The listing builds one solid part. Answer for the finished solid, in the listing's coordinates (mm). A direction names the side the tool comes from. Coordinates: 2 decimals unless noted, no trailing zeros. Order: outer loops, then holes, each group sorted by start corner. A loop starts at its lowest first (then second) coordinate and runs counter-clockwise, first axis right, second up. Notation, with made-up numbers: (43.25, 46.5) -> (90.25, 46.5) arc R19 cw to (90.25, 65.5) -> close; hole circle Ø2 at (20.5, 63.5). An arc over 180 degrees is marked (long way). Return JSON: item names as keys, results as strings.
Autodesk Inventor part; units mm, degrees
ref_plane "YZ Plane" through (0, 0, 0) normal (1, 0, 0) x (0, 1, 0)
ref_plane "XZ Plane" through (0, 0, 0) normal (0, 1, 0) x (-1, 0, 0)
ref_plane "XY Plane" through (0, 0, 0) normal (0, 0, 1) x (1, 0, 0)
sketch "Sketch1" plane through (0, 0, 0) normal (0, 1, 0) x (-1, 0, 0)
  line L0 (0, -14.7) -> (0, 14.7) construction
  line L1 (-13.4, 0) -> (33.15, 0) construction
  circle A0 centre (0, 0) radius 4.25
  circle A1 centre (16, 0) radius 7.975
  arc A2 (13.5391, -10.2075) -> (13.5391, 10.2075) centre (16, 0) ccw
  arc A3 (-1.582, 6.562) -> (-1.582, -6.562) centre (0, 0) ccw
  line L2 (13.5391, 10.2075) -> (-1.582, 6.562)
  line L3 (13.5391, -10.2075) -> (-1.582, -6.562)
  circle A4 centre (21, 0) radius 0.75
  circle A5 centre (11, 0) radius 0.75
  line L4 (16, 7.975) -> (16, -7.975) construction
  dimension "d0" = 8.5
  dimension "d1" = 15.95
  dimension "d2" = 16
  dimension "d3" = 21
  dimension "d4" = 13.5
  dimension "d5" = 1.5
  dimension "d6" = 1.5
  dimension "d7" = 10
extrude "Base" add sketch "Sketch1" along normal blind 3 contours A1 | L3 A3 L2 A2
extrude "Walls" add sketch "Sketch1" along normal blind 15 contours L3 A3 L2 A2
equation "\"d6\" = d5"
properties part number "transducer_holder" material "PC/ABS Plastic"
1. The part is cut by section B-B on x = -11. Give the vertices of the cut face in (y, z), and give its area (3 significant figures).
Answer block:
{"outline": "(0, -9.6) -> (15, -9.6) -> (15, -6.21) -> (3, -6.21) -> (3, -0.75) -> (0, -0.75) -> close; (0, 0.75) -> (3, 0.75) -> (3, 6.21) -> (15, 6.21) -> (15, 9.6) -> (0, 9.6) -> close", "area": "134 mm2"}
2. The part is cut by section C-C on y = 4.25. Give the number of separate pieces and of enclosed holes in the cut face, and give its area (3 significant figures).
Answer block:
{"separate pieces": "1", "enclosed holes": "2", "area": "272 mm2"}
3. Consider line 1 (X direction, y = 8.5, z = 3.5); line 2 (Z direction, x = -16, y = 11.75) (3 decimals); line 3 (X direction, y = 2.75, z = 3.75). Determine where each line is inside the solid, lowest interval first. Write a range as from..to.
Answer block:
{"line 1": "x = -25.9..-23.17, -8.83..-2.41, 2.41..5.77", "line 2": "z = -10.5..-7.975, 7.975..10.5", "line 3": "x = -25.81..-2, 2..5.61"}
4. For faces 1 (the face through (-26.497, 7.395, 0.266)), 2 (the face through (-16, 3, 0)), determine the directions among +Z, -Z, +X, -X, +Y, -Y from which every point of the face is accessible in a straight line to the end or side of a thin tool.
Answer block:
{"face 1": "+Y, -Y", "face 2": "+Y"}
5. Each of these flat-tipped pins is pushed along its axis until it touches: pin 1 Ø8 at (y, z) = (7.5, -0.5) entering from -X; pin 2 Ø3 at (x, y) = (-13, 2.5) entering from +Z; pin 3 Ø1.5 at (y, z) = (5.5, -7) entering from +X; pin 4 Ø1.5 at (x, y) = (-4.5, 8) entering from -Z. Where does it stop, or does it pass through?
Answer block:
{"pin 1": "stops at x = -26.5", "pin 2": "stops at z = 10.39", "pin 3": "stops at x = 2.55", "pin 4": "stops at z = -8.21"}
6. The part is cut by section A-A on z = 0. Give the vertices of the cut face in (x, y) (3 decimals).
Answer block:
{"outline": "(-26.5, 0) -> (-21.75, 0) -> (-21.75, 3) -> (-23.975, 3) -> (-23.975, 15) -> (-26.5, 15) -> close; (-20.25, 0) -> (-11.75, 0) -> (-11.75, 3) -> (-20.25, 3) -> close; (-10.25, 0) -> (-4.25, 0) -> (-4.25, 15) -> (-8.025, 15) -> (-8.025, 3) -> (-10.25, 3) -> close; (4.25, 0) -> (6.75, 0) -> (6.75, 15) -> (4.25, 15) -> close"}
7. The part is cut by section D-D on z = 2.5. Give the vertices of the cut face in (x, y), and give its area (3 significant figures).
Answer block:
{"outline": "(-26.2, 0) -> (-3.44, 0) -> (-3.44, 15) -> (-8.43, 15) -> (-8.43, 3) -> (-23.57, 3) -> (-23.57, 15) -> (-26.2, 15) -> close; (3.44, 0) -> (6.27, 0) -> (6.27, 15) -> (3.44, 15) -> close", "area": "202 mm2"}
8. Determine the mould class of faces 3 (the face through (-2.285, 7.395, -3.584)), 4 (the face through (-6, 15, 0)), 5 (the face through (6.75, 7.4, -0.13)) for opening direction X: pulls with the +X half, pulls with the -X half, needs draft (parallel to the pull), parting line crosses it, or undercut.
Answer block:
{"face 3": "undercut", "face 4": "needs draft", "face 5": "pulls with the +X half"}
